Build history of the part. All positions in model axes, mm. Face numbers are marked on the shaded views. A direction names the side the tool comes from. Coordinates: 2 decimals unless noted, no trailing zeros. Loops run counter-clockwise (first coordinate to the right, second up) from the corner with the lowest first, then second, coordinate; pieces in that order, holes last. Notation, with made-up numbers: (73, 85.25) - (130, 85.25) arc R34 cw to (130, 120.25) - close; hole circle Ø11 at (17, 22.5). An arc over 180 degrees is marked (long way). One line per item, written item: value.
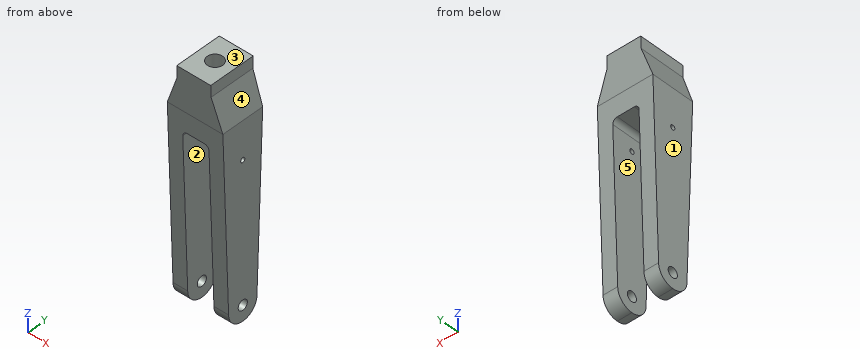
```python
from build123d import *

# Parameters (mm, degrees)
BOSS_EXTRUDE1_DEPTH = 30
SKETCH3_R           = 1.5
SKETCH3_R_2         = 3.25
CUT_EXTRUDE2_DEPTH  = 100
FILLET1_R           = 3
SKETCH6_R           = 5
CUT_EXTRUDE3_DEPTH  = 30


with BuildPart() as part:
    # Sketch1 → Boss-Extrude1 (new body)
    with BuildSketch(Plane(origin=(0, 0, 0), x_dir=(1, 0, 0), z_dir=(0, 1, 0))):
        Polygon((-7.001251561, 151.499010634), (2.498748439, 151.499010634), (2.498748439, 39.999010634), (19.498748439, 39.999010634), (19.498748439, 151.499010634), (28.998748439, 151.499010634), (28.998748439, 26.999010634), (21.998748439, 7.499010634), (21.998748439, -0.000989366), (-0.001251561, -0.000989366), (-0.001251561, 7.499010634), (-7.001251561, 26.999010634), align=None)
    extrude(amount=BOSS_EXTRUDE1_DEPTH)

    # Sketch3 → Cut-Extrude2 (cut)
    with BuildSketch(Plane(origin=(28.998748439, 0, 0), x_dir=(0, 0, -1), z_dir=(1, 0, 0))):
        with BuildLine():
            Line((26.999010634, 30), (26.999010634, 29.045936396))
            Line((26.999010634, 29.045936396), (141.499010634, 25))
            ThreePointArc((141.499010634, 25), (148.570078446, 22.071067812), (151.499010634, 15))
            Line((151.499010634, 15), (151.499010634, 30))
            Line((151.499010634, 30), (26.999010634, 30))
        make_face()
        with BuildLine():
            Line((141.499010634, 5), (26.999010634, 0.954063604))
            Line((26.999010634, 0.954063604), (26.999010634, 0))
            Line((26.999010634, 0), (151.499010634, 0))
            Line((151.499010634, 0), (151.499010634, 15))
            ThreePointArc((151.499010634, 15), (148.570078446, 7.928932188), (141.499010634, 5))
        make_face()
        Polygon((26.999010634, 30), (-0.000989366, 30), (26.999010634, 29.045936396), align=None)
        Polygon((26.999010634, 0.954063604), (-0.000989366, 0), (26.999010634, 0), align=None)
        with Locations((51.499010634, 15)):
            Circle(SKETCH3_R)
        with Locations((141.499010634, 15)):
            Circle(SKETCH3_R_2)
    extrude(amount=-CUT_EXTRUDE2_DEPTH, mode=Mode.SUBTRACT)

    # Fillet1
    fillet1_edges = [part.edges().sort_by_distance(p)[0] for p in [
        (2.498748439, 15, -39.999010634),
        (19.498748439, 15, -39.999010634),
    ]]
    fillet(fillet1_edges, radius=FILLET1_R)

    # Sketch6 → Cut-Extrude3 (cut)
    with BuildSketch(Plane.XY.offset(0.000989366)):
        with Locations((10.998748439, 15)):
            Circle(SKETCH6_R)
    extrude(amount=-CUT_EXTRUDE3_DEPTH, mode=Mode.SUBTRACT)


solid = part.part
```
Item 1: Cut at D-D, the plane y = 22. Write the cut outline in (x, z), then the cut area to 3 significant figures.
Check result:
outline: (-7, -148.64) - (2.5, -148.64) - (2.5, -43) arc R3 cw to (5.5, -40) - (16.5, -40) arc R3 cw to (19.5, -43) - (19.5, -148.64) - (29, -148.64) - (29, -27) - (22, -7.5) - (22, 0) - (0, 0) - (0, -7.5) - (-7, -27) - close
area: 3,270 mm^2
Item 2: Probe probe 1 along X at (y, z) = (17.5, -60.5); probe 2 along Z at (x, y) = (7, 7); probe 3 along X at (y, z) = (16.5, -40.5). List the from-to ranges inside material, lowest first. Write a range as from..to.
Check result:
probe 1: x = -7..2.5, 19.5..29
probe 2: z = -40..0
probe 3: x = -7..3.84, 18.16..29
Item 3: Cut at A-A, the plane z = -109. Write the cut outline in (x, y).
Check result:
outline: (-7, 3.85) - (2.5, 3.85) - (2.5, 26.15) - (-7, 26.15) - close; (19.5, 3.85) - (29, 3.85) - (29, 26.15) - (19.5, 26.15) - close
Item 4: Cut at B-B, the plane x = -4. Write the cut outline in (y, z), then the cut area to 3 significant figures.
Check result:
outline: (0.66, -18.64) - (5, -141.5) arc R10 ccw to (25, -141.5) - (29.34, -18.64) - close; hole circle Ø6.5 at (15, -141.5); hole circle Ø3 at (15, -51.5)
area: 3,110 mm^2
Item 5: Cut at C-C, the plane z = -24. Write the cut outline in (x, y).
Check result:
outline: (-5.92, 0.85) - (27.92, 0.85) - (27.92, 29.15) - (-5.92, 29.15) - close; hole circle Ø10 at (11, 15)
Item 6: Tool access for the marked faces 1 and 2: list every direction of +Z, -Z, +X, -X, +Y, -Y with a clear straight run to the whole face (end or side of a thin tool).
Check result:
face 1: +Z, -Z, -X, +Y, -Y
face 2: -Z, +Y, -Y
Item 7: Drop flat-ended pins along their axis: P1, Ø5, axis at y = 15, z = -51.5, coming from the +X side; P2, Ø3, axis at x = 10.5, y = 16.5, coming from the +Z side; P3, Ø2, axis at x = 7.5, y = 27, coming from the -Z side; P4, Ø6, axis at y = 18.5, z = -2.5, coming from the -X side. Give the stop position or say it passes through.
Check result:
P1: stops at x = 29
P2: stops at z = -30
P3: stops at z = -40
P4: stops at x = 0
Item 8: Pull direction X, two halves, no side cores. Call the marked faces 3, 4 and 5: released by +X, released by -X, zero draft, split by the parting line, or undercut.
Check result:
face 3: zero draft
face 4: released by +X
face 5: undercut
